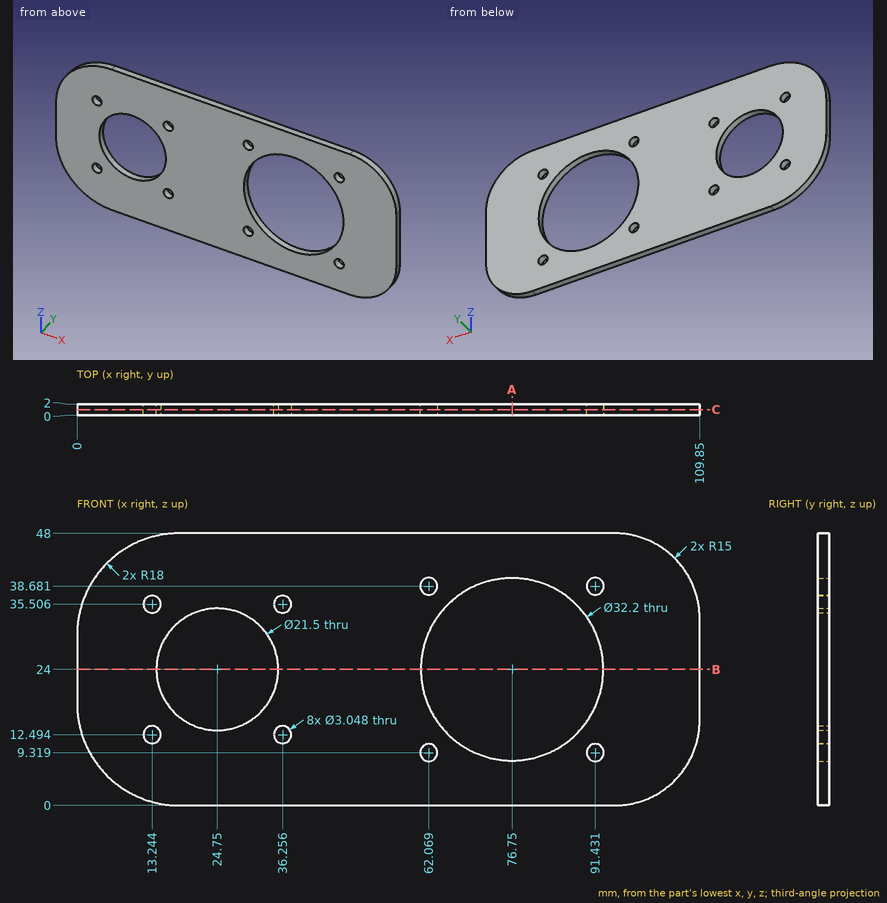
Drawing for the job (mm, zero at the part's lowest x, y, z). Give positions to 0.01 mm unless a question says otherwise; leave off trailing zeros. Order: outer loops, then holes, each group sorted by start corner. A loop starts at its lowest first (then second) coordinate and runs counter-clockwise, first axis right, second up. Notation, with made-up numbers: M -37.5,48.5 L -24.5,48.5 A30 ccw -24.5,71.5 Z; hole C 73.5,-6 d7. An arc over 180 degrees is marked long. Use a Markdown table: item, result. Add a question column.
(1) Probe line 1 along Z through (x, y) = (36.5, 1.25); line 2 along X through (y, z) = (0.7, 12.5); line 3 along X through (y, z) = (1.8, 13) (1 decimal). List the from-to ranges inside material, lowest first. Write a range as [from, to].
(2) Saw through at B-B, the plane z = 24. Give the cut face in (x, y), and give its area (3 significant figures).
(3) Saw through at A-A, the plane x = 76.75. Give the cut face in (y, z), and give its area (3 significant figures).
(4) Saw through at C-C, the plane y = 1. Give the number of separate pieces and of enclosed holes in the cut face, and give its area (3 significant figures).
(5) Drop flat-ended pins along their axis: P1, Ø3.5, axis at x = 62.07, z = 9.32, coming from the -Y side; P2, Ø1, axis at y = 1, z = 32, coming from the -X side. Give the stop position or say it passes through.
Answer key:
| question | item | result |
|---|---|---|
| 1 | line 1 | [0, 10.99], [14, 34], [37.01, 48] |
| 1 | line 2 | [0.86, 11.72], [14.77, 34.73], [37.78, 65.48], [88.02, 109.64] |
| 1 | line 3 | [0.7, 11.8], [14.7, 34.8], [37.7, 65], [88.5, 109.7] |
| 2 | outline | M 0,0 L 14,0 L 14,2 L 0,2 Z; M 35.5,0 L 60.65,0 L 60.65,2 L 35.5,2 Z; M 92.85,0 L 109.85,0 L 109.85,2 L 92.85,2 Z |
| 2 | area | 112 mm^2 |
| 3 | outline | M 0,0 L 2,0 L 2,7.9 L 0,7.9 Z; M 0,40.1 L 2,40.1 L 2,48 L 0,48 Z |
| 3 | area | 31.6 mm^2 |
| 4 | separate pieces | 1 |
| 4 | enclosed holes | 10 |
| 4 | area | 3,800 mm^2 |
| 5 | P1 | y = 0 |
| 5 | P2 | x = 0.06 |
